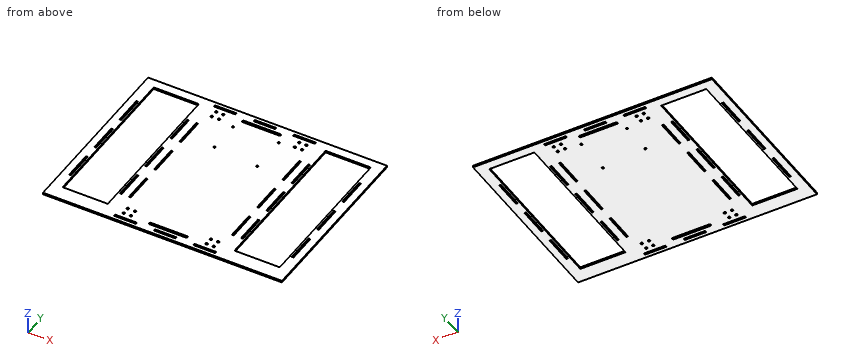
from build123d import *

# Parameters (mm, degrees)
F0_R     = 1.984375
F0_W     = 38.1
F0_H     = 3.302
F0_W_2   = 3.302
F0_H_2   = 50.8
F0_W_3   = 79.248
F0_H_3   = 275.232702
F0_R_2   = 1.75
F1_DEPTH = 3.175


with BuildPart() as f1:
    # F0 (on Top) → F1 (new body)
    with BuildSketch(Plane.XY):
        Polygon((-111.125, -158.75), (111.125, -158.75), (209.55, -158.75), (209.55, 158.75), (111.125, 158.75), (-111.125, 158.75), (-209.55, 158.75), (-209.55, -158.75), align=None)
        with Locations((-79.121, -139.573)):
            Circle(F0_R, mode=Mode.SUBTRACT)
        with Locations((-69.596, -150.749)):
            Rectangle(F0_W, F0_H, mode=Mode.SUBTRACT)
        with Locations((-66.421, -139.573)):
            Circle(F0_R, mode=Mode.SUBTRACT)
        with Locations((-79.121, -126.873)):
            Circle(F0_R, mode=Mode.SUBTRACT)
        with Locations((-66.421, -126.873)):
            Circle(F0_R, mode=Mode.SUBTRACT)
        with Locations((-195.199, -76.2)):
            Rectangle(F0_W_2, F0_H_2, mode=Mode.SUBTRACT)
        with Locations((-106.299, -76.2)):
            Rectangle(F0_W_2, F0_H_2, mode=Mode.SUBTRACT)
        with Locations((-90.297, -76.2)):
            Rectangle(F0_W_2, F0_H_2, mode=Mode.SUBTRACT)
        with Locations((0, -150.749)):
            Rectangle(F0_W, F0_H, mode=Mode.SUBTRACT)
        with BuildLine():
            ThreePointArc((-31.75, -142.748), (-33.734375, -140.763625), (-31.75, -138.77925))
            Line((-31.75, -138.77925), (0, -138.77925))
            Line((0, -138.77925), (31.75, -138.77925))
            ThreePointArc((31.75, -138.77925), (33.734375, -140.763625), (31.75, -142.748))
            Line((31.75, -142.748), (0, -142.748))
            Line((0, -142.748), (-31.75, -142.748))
        make_face(mode=Mode.SUBTRACT)
        with Locations((69.596, -150.749)):
            Rectangle(F0_W, F0_H, mode=Mode.SUBTRACT)
        with Locations((66.421, -139.573)):
            Circle(F0_R, mode=Mode.SUBTRACT)
        with Locations((79.121, -139.573)):
            Circle(F0_R, mode=Mode.SUBTRACT)
        with Locations((66.421, -126.873)):
            Circle(F0_R, mode=Mode.SUBTRACT)
        with Locations((79.121, -126.873)):
            Circle(F0_R, mode=Mode.SUBTRACT)
        with Locations((90.297, -76.2)):
            Rectangle(F0_W_2, F0_H_2, mode=Mode.SUBTRACT)
        with Locations((106.299, -76.2)):
            Rectangle(F0_W_2, F0_H_2, mode=Mode.SUBTRACT)
        with Locations((195.199, -76.2)):
            Rectangle(F0_W_2, F0_H_2, mode=Mode.SUBTRACT)
        with Locations((-195.199, 0)):
            Rectangle(F0_W_2, F0_H_2, mode=Mode.SUBTRACT)
        with Locations((-150.749, 5.131649)):
            Rectangle(F0_W_3, F0_H_3, mode=Mode.SUBTRACT)
        with Locations((-106.299, 0)):
            Rectangle(F0_W_2, F0_H_2, mode=Mode.SUBTRACT)
        with Locations((-195.199, 76.2)):
            Rectangle(F0_W_2, F0_H_2, mode=Mode.SUBTRACT)
        with Locations((-106.299, 76.2)):
            Rectangle(F0_W_2, F0_H_2, mode=Mode.SUBTRACT)
        with Locations((-90.297, 0)):
            Rectangle(F0_W_2, F0_H_2, mode=Mode.SUBTRACT)
        with Locations((-90.297, 76.2)):
            Rectangle(F0_W_2, F0_H_2, mode=Mode.SUBTRACT)
        with Locations((-39.037, 65.881)):
            Circle(F0_R_2, mode=Mode.SUBTRACT)
        with Locations((-79.121, 126.873)):
            Circle(F0_R, mode=Mode.SUBTRACT)
        with Locations((-66.421, 126.873)):
            Circle(F0_R, mode=Mode.SUBTRACT)
        with Locations((-79.121, 139.573)):
            Circle(F0_R, mode=Mode.SUBTRACT)
        with Locations((-66.421, 139.573)):
            Circle(F0_R, mode=Mode.SUBTRACT)
        with Locations((-69.596, 150.749)):
            Rectangle(F0_W, F0_H, mode=Mode.SUBTRACT)
        with Locations((-39.037, 121.615)):
            Circle(F0_R_2, mode=Mode.SUBTRACT)
        with Locations((90.297, 0)):
            Rectangle(F0_W_2, F0_H_2, mode=Mode.SUBTRACT)
        with Locations((39.921, 58.698)):
            Circle(F0_R_2, mode=Mode.SUBTRACT)
        with Locations((90.297, 76.2)):
            Rectangle(F0_W_2, F0_H_2, mode=Mode.SUBTRACT)
        with Locations((106.299, 0)):
            Rectangle(F0_W_2, F0_H_2, mode=Mode.SUBTRACT)
        with Locations((150.749, 5.131649)):
            Rectangle(F0_W_3, F0_H_3, mode=Mode.SUBTRACT)
        with Locations((195.199, 0)):
            Rectangle(F0_W_2, F0_H_2, mode=Mode.SUBTRACT)
        with Locations((106.299, 76.2)):
            Rectangle(F0_W_2, F0_H_2, mode=Mode.SUBTRACT)
        with Locations((195.199, 76.2)):
            Rectangle(F0_W_2, F0_H_2, mode=Mode.SUBTRACT)
        with Locations((39.921, 123.698)):
            Circle(F0_R_2, mode=Mode.SUBTRACT)
        with BuildLine():
            Line((-31.75, 142.748), (0, 142.748))
            Line((0, 142.748), (31.75, 142.748))
            ThreePointArc((31.75, 142.748), (33.734375, 140.763625), (31.75, 138.77925))
            Line((31.75, 138.77925), (0, 138.77925))
            Line((0, 138.77925), (-31.75, 138.77925))
            ThreePointArc((-31.75, 138.77925), (-33.734375, 140.763625), (-31.75, 142.748))
        make_face(mode=Mode.SUBTRACT)
        with Locations((0, 150.749)):
            Rectangle(F0_W, F0_H, mode=Mode.SUBTRACT)
        with Locations((66.421, 126.873)):
            Circle(F0_R, mode=Mode.SUBTRACT)
        with Locations((79.121, 126.873)):
            Circle(F0_R, mode=Mode.SUBTRACT)
        with Locations((66.421, 139.573)):
            Circle(F0_R, mode=Mode.SUBTRACT)
        with Locations((69.596, 150.749)):
            Rectangle(F0_W, F0_H, mode=Mode.SUBTRACT)
        with Locations((79.121, 139.573)):
            Circle(F0_R, mode=Mode.SUBTRACT)
    extrude(amount=F1_DEPTH)


solid = f1.part
Geometry check sheet. Reference: the model listing, model coordinates, mm. Coordinates: 2 decimals unless noted, no trailing zeros. Order: outer loops, then holes, each group sorted by start corner. A loop starts at its lowest first (then second) coordinate and runs counter-clockwise, first axis right, second up. Notation, with made-up numbers: (76, -38.5) - (119, -38.5) arc R23 ccw to (119, -19.5) - close; hole circle Ø10 at (59.25, 69.5). An arc over 180 degrees is marked (long way). One line per item, written item: value.
(1) Thickness scan on probe 1 along Y at (x, z) = (-85, 1.3); probe 2 along Y at (x, z) = (-1.5, 2.2); probe 3 along X at (y, z) = (131.5, 1.1) (3 decimals). Record the ranges inside material, lowest first. Write a range as from..to.
Data:
probe 1: y = -158.75..-152.4, -149.1..149.1, 152.4..158.75
probe 2: y = -158.75..-152.4, -149.1..-142.75, -138.78..138.78, 142.75..149.1, 152.4..158.75
probe 3: x = -209.55..-190.373, -111.125..111.125, 190.373..209.55
(2) Sectioned sample at C-C (z = 1.3). Count the separate pieces of the cut face and the enclosed holes in it, and give its area (3 significant figures).
Data:
separate pieces: 1
enclosed holes: 48
area: 84,900 mm^2
(3) Depth check by flat-ended pin: pin 1 Ø3.5 at (x, y) = (66.421, 126.873) entering from -Z. Enter the tip coordinate at first touch or a pass-through.
Data:
pin 1: passes through
(4) Sectioned sample at B-B (y = 34). Enter the section's corners in (x, z) (3 decimals), and give its area (3 significant figures).
Data:
outline: (-209.55, 0) - (-190.373, 0) - (-190.373, 3.175) - (-209.55, 3.175) - close; (-111.125, 0) - (111.125, 0) - (111.125, 3.175) - (-111.125, 3.175) - close; (190.373, 0) - (209.55, 0) - (209.55, 3.175) - (190.373, 3.175) - close
area: 827 mm^2
(5) Sectioned sample at A-A (x = 140). Enter the section's corners in (y, z) (3 decimals), and give its area (3 significant figures).
Data:
outline: (-158.75, 0) - (-132.485, 0) - (-132.485, 3.175) - (-158.75, 3.175) - close; (142.748, 0) - (158.75, 0) - (158.75, 3.175) - (142.748, 3.175) - close
area: 134 mm^2
